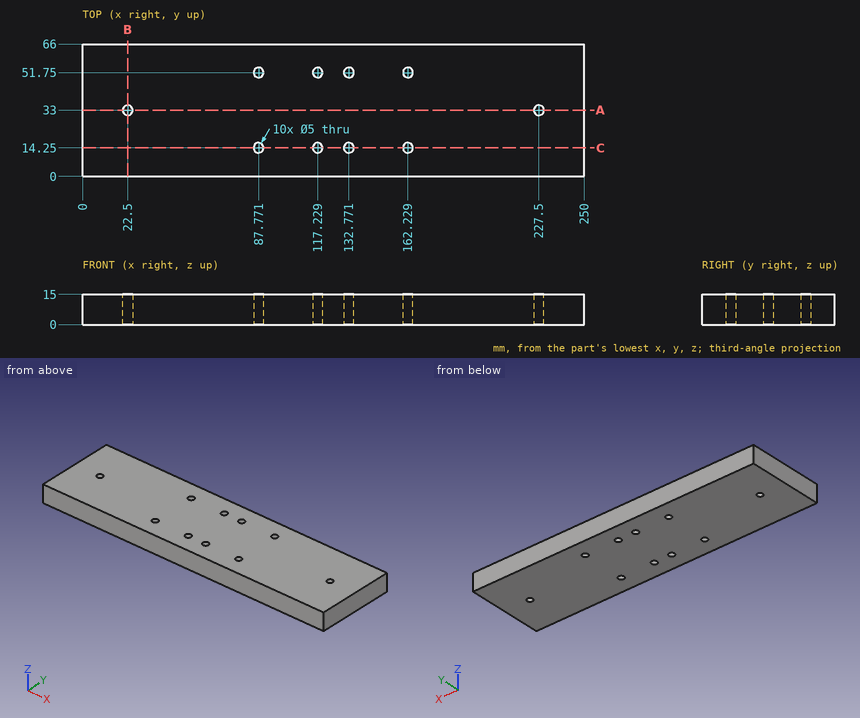
Source: three-view drawing plus pictorial views. Frame: mm from the lowest corner of the part. Give positions to 0.01 mm unless a question says otherwise; leave off trailing zeros. Write each loop counter-clockwise with the first axis right and the second up, starting at its lowest first coordinate (ties: lowest second). Pieces come first, ordered by that corner, then holes. Notation, with made-up numbers: (15.25, 3.25) -> (47.25, 3.25) arc R13 ccw to (47.25, 10.25) -> close; hole circle Ø2 at (1.25, -15.75). An arc over 180 degrees is marked (long way). Write item = value, one per line.
Q1. First-contact query: pin 1 (4.5 mm diameter, centred on x = 87.77, y = 51.75, fed in from -Z). Flat tip, straight axial feed; report the tip coordinate or a pass-through.
Here are the results:
pin_1 = through
Q2. Line query: line 1 (Y direction, x = 22.5, z = 8.25); line 2 (Y direction, x = 116, z = 5.5); line 3 (X direction, y = 35, z = 1.75). Output: solid intervals per line, ascending. Write a range as from..to.
Here are the results:
line_1 = 0..30.5, 35.5..66
line_2 = 0..12.07, 16.43..49.57, 53.93..66
line_3 = 0..21, 24..226, 229..250
Q3. Cut plane A-A on y = 33. Return loops of the section in (x, z), then the cut area to 3 significant figures.
Here are the results:
outline = (0, 0) -> (20, 0) -> (20, 15) -> (0, 15) -> close; (25, 0) -> (225, 0) -> (225, 15) -> (25, 15) -> close; (230, 0) -> (250, 0) -> (250, 15) -> (230, 15) -> close
area = 3,600 mm²
Q4. Cut plane C-C on y = 14.25. Return loops of the section in (x, z).
Here are the results:
outline = (0, 0) -> (85.27, 0) -> (85.27, 15) -> (0, 15) -> close; (90.27, 0) -> (114.73, 0) -> (114.73, 15) -> (90.27, 15) -> close; (119.73, 0) -> (130.27, 0) -> (130.27, 15) -> (119.73, 15) -> close; (135.27, 0) -> (159.73, 0) -> (159.73, 15) -> (135.27, 15) -> close; (164.73, 0) -> (250, 0) -> (250, 15) -> (164.73, 15) -> close
Q5. Cut plane B-B on x = 22.5. Return loops of the section in (y, z).
Here are the results:
outline = (0, 0) -> (30.5, 0) -> (30.5, 15) -> (0, 15) -> close; (35.5, 0) -> (66, 0) -> (66, 15) -> (35.5, 15) -> close
